Geometry: final body of the model. Coordinates: model frame, mm. Coordinates: 2 decimals unless noted, no trailing zeros. Order: outer loops, then holes, each group sorted by start corner. A loop starts at its lowest first (then second) coordinate and runs counter-clockwise, first axis right, second up. Notation, with made-up numbers: (-32.75, 11) -> (-2.75, 11) arc R25 cw to (-2.75, 49) -> close; hole circle Ø2 at (-11, -23.75). An arc over 180 degrees is marked (long way). Use one line per item in the form item = value.
```python
from build123d import *

# Parameters (mm, degrees)
F0_R        = 10
F1_DEPTH    = 25
F2_DEPTH    = 50
F3_T4_ANGLE = 203.6133668192
F3_T6_ANGLE = 179.9906971182


# Not quite as in the source:
# - a fillet or chamfer that OpenCascade refuses, or shapes differently, is made with other operations: its cross-section is extruded or revolved along the edge and cut away or added


with BuildPart() as f1:
    # F0 (on Front) → F1 (new body)
    with BuildSketch(Plane.XZ):
        with BuildLine():
            Line((2.8107571296, 24.8414903812), (0, 25))
            ThreePointArc((0, 25), (-25, 0), (0, -25))
            Line((0, -25), (2.8107571296, -24.8414903812))
            ThreePointArc((2.8107571296, -24.8414903812), (18.6449581421, -16.6542948179), (25, 0))
            ThreePointArc((25, 0), (18.6449581421, 16.6542948179), (2.8107571296, 24.8414903812))
        make_face()
        Circle(F0_R, mode=Mode.SUBTRACT)
        with BuildLine():
            ThreePointArc((2.8107571296, 24.8414903812), (1.4076115356, 24.9603411388), (0, 25))
            Line((0, 25), (2.8107571296, 24.8414903812))
        make_face()
        with BuildLine():
            Line((2.8107571296, -24.8414903812), (0, -25))
            ThreePointArc((0, -25), (1.4076115356, -24.9603411388), (2.8107571296, -24.8414903812))
        make_face()
        with BuildLine():
            Line((133.4853280749, 17.4722387972), (2.8107571296, 24.8414903812))
            ThreePointArc((2.8107571296, 24.8414903812), (18.6449581421, 16.6542948179), (25, 0))
            ThreePointArc((25, 0), (18.6449581421, -16.6542948179), (2.8107571296, -24.8414903812))
            Line((2.8107571296, -24.8414903812), (133.4853280749, -17.4722387972))
            ThreePointArc((133.4853280749, -17.4722387972), (115, 0), (133.4853280749, 17.4722387972))
        make_face()
        with BuildLine():
            ThreePointArc((150, 0), (145.2179644855, 12.0209558415), (133.4853280749, 17.4722387972))
            ThreePointArc((133.4853280749, 17.4722387972), (115, 0), (133.4853280749, -17.4722387972))
            ThreePointArc((133.4853280749, -17.4722387972), (145.2179644855, -12.0209558415), (150, 0))
        make_face()
        with Locations((132.5, 0)):
            Circle(F0_R, mode=Mode.SUBTRACT)
    extrude(amount=F1_DEPTH)

    # F0 (on Front) → F2 (join)
    with BuildSketch(Plane.XZ):
        with BuildLine():
            Line((2.8107571296, 24.8414903812), (0, 25))
            ThreePointArc((0, 25), (-25, 0), (0, -25))
            Line((0, -25), (2.8107571296, -24.8414903812))
            ThreePointArc((2.8107571296, -24.8414903812), (18.6449581421, -16.6542948179), (25, 0))
            ThreePointArc((25, 0), (18.6449581421, 16.6542948179), (2.8107571296, 24.8414903812))
        make_face()
        Circle(F0_R, mode=Mode.SUBTRACT)
    extrude(amount=F2_DEPTH)

    # F3: chamfer of 2 on 4 edges, made by hand

    # F3_s1 → F3_t2 (revolve, cut)
    with BuildSketch(Plane.XY):
        Polygon((12, -50), (10, -48), (10, -50), align=None)
    revolve(axis=Axis((0, -50, 0), (0, -1, 0)), mode=Mode.SUBTRACT)

    # F3_s3 → F3_t4 (revolve, cut)
    with BuildSketch(Plane(origin=(0, 0, 0), x_dir=(0, 1, 0), z_dir=(0.9788435281, 0, -0.2046102329))):
        Polygon((-48, 25), (-50, 23), (-50, 25), align=None)
    revolve(axis=Axis((0, -50, 0), (0, -1, 0)), revolution_arc=F3_T4_ANGLE, mode=Mode.SUBTRACT)

    # F3_s5 → F3_t6 (revolve, cut)
    with BuildSketch(Plane(origin=(0, 0, 0), x_dir=(0, 1, 0), z_dir=(-0.9999999967, 0, 8.1183e-05))):
        Polygon((-48, -25), (-50, -23), (-50, -25), align=None)
    revolve(axis=Axis((0, -50, 0), (0, 1, 0)), revolution_arc=F3_T6_ANGLE, mode=Mode.SUBTRACT)

    # F3_s7 → F3_t8 (revolve, cut)
    with BuildSketch(Plane.XY):
        Polygon((144.5, -25), (142.5, -23), (142.5, -25), align=None)
    revolve(axis=Axis((132.5, -25, 0), (0, -1, 0)), mode=Mode.SUBTRACT)


solid = f1.part
```
1) Section C-C, the plane x = 102.5. Output: boundary loops of the cut face in (y, z), and give its area (3 significant figures).
Results found:
outline = (-25, -19.22) -> (0, -19.22) -> (0, 19.22) -> (-25, 19.22) -> close
area = 961 mm2
2) Material intervals for probe 1 along Z at (x, y) = (0, -22); probe 2 along X at (y, z) = (-12.5, -8); probe 3 along Y at (x, z) = (61, -19), sorted ascending. Write a range as from..to.
Results found:
probe_1 = -25..-10, 10..25
probe_2 = -23.69..-6, 6..126.5, 138.5..148.06
probe_3 = -25..0
3) Section A-A, the plane y = -42.5. Output: boundary loops of the cut face in (x, z), and give its area (3 significant figures).
Results found:
outline = (0, -25) -> (2.81, -24.84) arc R25 ccw to (2.81, 24.84) -> (0, 25) arc R25 ccw to start; hole circle Ø20 at (0, 0)
area = 1,650 mm2
4) Section B-B, the plane z = -3.5. Give the number of separate pieces and of enclosed holes in the cut face, and give its area (3 significant figures).
Results found:
separate_pieces = 3
enclosed_holes = 0
area = 4,180 mm2
5) Pull-direction query (X, two-part tool) for faces 1 (the flat face through (67.23, -12.32, -21.21)), 2 (the flat face through (61, 0, 0)), 3 (the cylindrical face through (-2.17, -23.66, -9.76)); classes: released by +X, released by -X, zero draft, split by the parting line, or undercut.
Results found:
face_1 = released by +X
face_2 = zero draft
face_3 = undercut
6) Contact query for flat-ended pins moving along their axis: P1, Ø10, axis at x = 96.5, z = 14, coming from the -Y side; P2, Ø1, axis at x = 131.5, y = -13, coming from the +Z side; P3, Ø10, axis at x = 42.5, y = -22.5, coming from the -Z side. Output: stop coordinate, or through.
Results found:
P1 = -25
P2 = 17.61
P3 = -22.89
